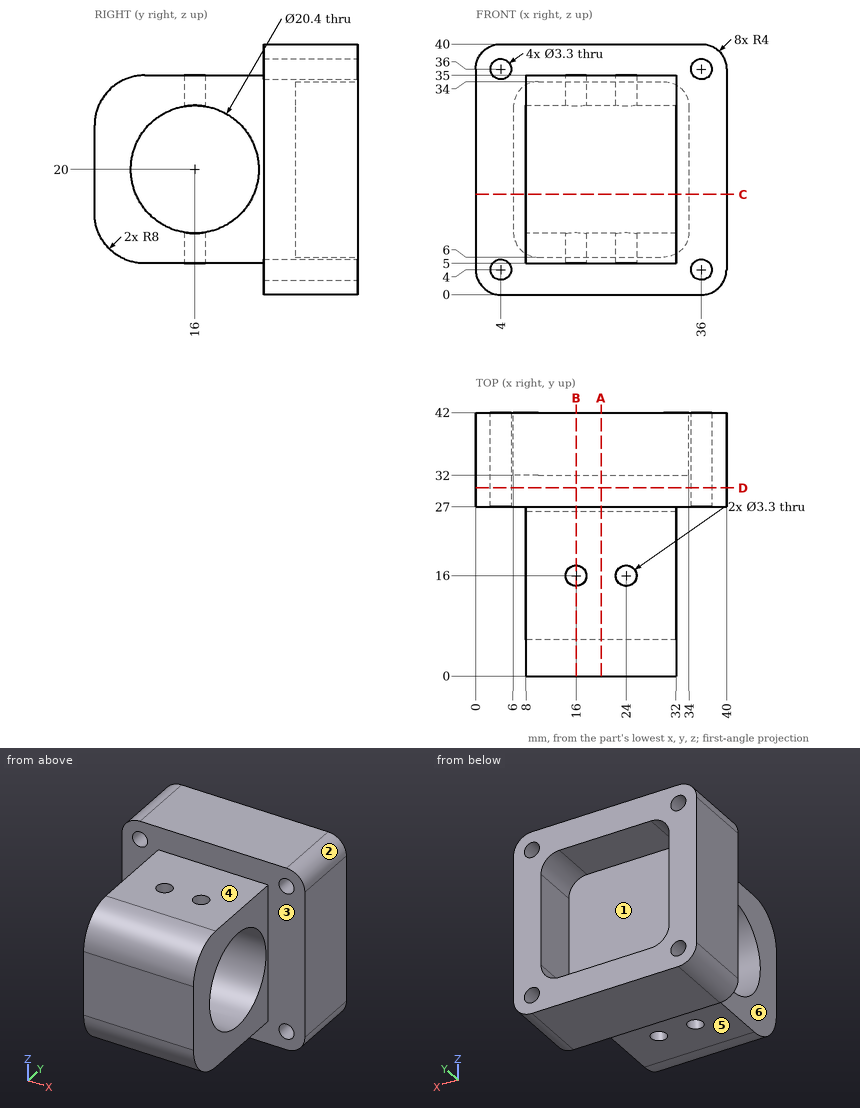
For this review, use the dimensioned drawing (mm, ordinates from the lowest corner) and the shaded views. A direction names the side the tool comes from. Coordinates: 2 decimals unless noted, no trailing zeros. Order: outer loops, then holes, each group sorted by start corner. A loop starts at its lowest first (then second) coordinate and runs counter-clockwise, first axis right, second up. Notation, with made-up numbers: (-28, 22) - (-5, 22) arc R11 cw to (-5, 41) - close; hole circle Ø9 at (87.5, 29). An arc over 180 degrees is marked (long way). Answer as a JSON object with one key per item and string values. Group by question number.
1. We need section C-C on z = 16. State the section outline as (x, y) points.
2. The part is to be moulded in two halves that separate along X. For the marked faces 1, 2 and 3, say which applies: pulls with the +X half, pulls with the -X half, needs draft (parallel to the pull), parting line crosses it, or undercut.
3. We need section A-A on x = 20. State the section outline as (y, z) points.
4. Clearance check with flat-ended pins moving along their axes: P1, Ø4, axis at x = 16, y = 16, coming from the +Z side; P2, Ø1.5, axis at y = 8, z = 31, coming from the -X side; P3, Ø1.5, axis at x = 23, y = 8, coming from the -Z side. State where each tip first meets the part, or that it passes through.
5. We need section B-B on x = 16. State the section outline as (y, z) points, then the cut area to 3 significant figures.
6. For the marked faces 4, 5 and 6, list the 3-axis set-ups (+Z, -Z, +X, -X, +Y, -Y) from which the entire face can be reached by the end or side of a thin tool; tool diameter is ignored.
7. We need section D-D on y = 30. State the section outline as (x, z) points.
8. For probe 1 along X at (y, z) = (16, 7.7); probe 2 along Z at (x, y) = (4, 30.75), list the stretches that pass through material, from the lowest coordinate up.
Final values:
{
 "1": {"outline": "(0, 27) - (8, 27) - (8, 25.38) - (32, 25.38) - (32, 27) - (40, 27) - (40, 42) - (34, 42) - (34, 32) - (6, 32) - (6, 42) - (0, 42) - close; (8, 0) - (32, 0) - (32, 6.62) - (8, 6.62) - close"},
 "2": {"face 1": "undercut", "face 2": "pulls with the +X half", "face 3": "needs draft"},
 "3": {"outline": "(0, 13) arc R8 ccw to (8, 5) - (27, 5) - (27, 0) - (42, 0) - (42, 6) - (32, 6) - (32, 34) - (42, 34) - (42, 40) - (27, 40) - (27, 35) - (8, 35) arc R8 ccw to (0, 27) - close; hole circle Ø20.4 at (16, 20)"},
 "4": {"P1": "z = 35", "P2": "x = 8", "P3": "z = 5"},
 "5": {"outline": "(0, 13) arc R8 ccw to (8, 5) - (14.35, 5) - (14.35, 9.93) arc R10.2 cw to (14.35, 30.07) - (14.35, 35) - (8, 35) arc R8 ccw to (0, 27) - close; (17.65, 5) - (27, 5) - (27, 0) - (42, 0) - (42, 6) - (32, 6) - (32, 34) - (42, 34) - (42, 40) - (27, 40) - (27, 35) - (17.65, 35) - (17.65, 30.07) arc R10.2 cw to (17.65, 9.93) - close", "area": "744 mm²"},
 "6": {"face 4": "+Z, +X, -X, -Y", "face 5": "-Z, +X, -X, -Y", "face 6": "+Z, -Z, -X, -Y"},
 "7": {"outline": "(0, 4) arc R4 ccw to (4, 0) - (36, 0) arc R4 ccw to (40, 4) - (40, 36) arc R4 ccw to (36, 40) - (4, 40) arc R4 ccw to (0, 36) - close; hole circle Ø3.3 at (4, 4); hole circle Ø3.3 at (4, 36); hole circle Ø3.3 at (36, 4); hole circle Ø3.3 at (36, 36)"},
 "8": {"probe 1": "8 to 14.35, 17.65 to 22.35, 25.65 to 32", "probe 2": "0 to 2.35, 5.65 to 34.35, 37.65 to 40"}
}
